```python
from build123d import *

# Parameters (mm, degrees)
F1_DEPTH = 3.175
F2_R     = 2.54
F3_DEPTH = 12.7
F4_R     = 1.1938
F5_DEPTH = 2.54


with BuildPart() as f1:
    # F0 (on Top) → F1 (new body)
    with BuildSketch(Plane.XY):
        with BuildLine():
            Line((32.885008, 3.175), (0, 3.175))
            ThreePointArc((0, 3.175), (-3.175, 0), (0, -3.175))
            Line((0, -3.175), (32.885008, -3.175))
            ThreePointArc((32.885008, -3.175), (36.060008, 0), (32.885008, 3.175))
        make_face()
    extrude(amount=F1_DEPTH)

    # F2 (on face) → F3 (join)
    with BuildSketch(Plane.XY.offset(3.175)):
        with Locations((1.6764, 0)):
            Circle(F2_R)
    extrude(amount=F3_DEPTH)

    # F4 (on face) → F5 (join)
    with BuildSketch(Plane(origin=(0, 0, 0), x_dir=(1, 0, 0), z_dir=(0, 0, -1))):
        with Locations((13.335, 0)):
            Circle(F4_R)
        with Locations((29.845, 0)):
            Circle(F4_R)
    extrude(amount=F5_DEPTH)


solid = f1.part
```
Design review of the part built by this model. Coordinates are the model's own, in mm. A direction names the side the tool comes from. Give positions to 0.01 mm unless a question says otherwise; leave off trailing zeros. Loops run counter-clockwise (first coordinate to the right, second up) from the corner with the lowest first, then second, coordinate; pieces in that order, holes last. Notation, with made-up numbers: M 23.5,24 L 39.5,24 A23 ccw 39.5,37 Z; hole C 60.25,-4.75 d9. An arc over 180 degrees is marked long. Return JSON: item names as keys, results as strings. Group by question number.
Item 1: Mouldability with a two-part tool opening along X and no side actions: class faces 4 (the cylindrical face through (-3.174, 0.07, 1.565)), 5 (the flat face through (2, 0, 15.875)), 6 (the cylindrical face through (36.06, -0.07, 1.57)), 7 (the cylindrical face through (12.142, -0.052, -1.252)) as released by +X, released by -X, zero draft, split by the parting line, or undercut.
Item 2: We need section A-A (y = 0). Give the boundary of the cut face in (x, z) (3 decimals).
Item 3: Insertion check: pin 1 Ø1 at (y, z) = (1, 7.5) entering from +X; pin 2 Ø1 at (x, y) = (16, 0) entering from -Z; pin 3 Ø2 at (y, z) = (1.5, 7.5) entering from -X; pin 4 Ø1.5 at (x, z) = (7.5, 4) entering from +Y. Each pin has a flat end and moves straight along its axis. Give the tip position at first contact, or say it passes through.
Item 4: Tool access review of faces 1 (the cylindrical face through (4.1, 0.76, 9.44)), 2 (the cylindrical face through (30.984, -0.359, -1.252)), 3 (the flat face through (17, 3.175, 2)): name each direction out of +Z, -Z, +X, -X, +Y, -Y from which nothing blocks a thin tool from reaching the whole face with its end or side.
Item 5: We need section B-B (z = 14.25). Give the boundary of the cut face in (x, y).
Item 6: We need section D-D (y = 2). Give the boundary of the cut face in (x, z) (3 decimals).
Item 7: For probe 1 along X at (y, z) = (0, -1.5); probe 2 along Z at (x, y) = (8, 1.75) (3 decimals); probe 3 along Z at (x, y) = (2, -1.25) (3 decimals), list the stretches that pass through material, from the lowest coordinate up.
Item 8: We need section C-C (x = 8.5). Give the boundary of the cut face in (y, z) (3 decimals).
Output:
{
 "1": {"face 4": "released by -X", "face 5": "zero draft", "face 6": "released by +X", "face 7": "undercut"},
 "2": {"outline": "M -3.175,0 L 12.141,0 L 12.141,-2.54 L 14.529,-2.54 L 14.529,0 L 28.651,0 L 28.651,-2.54 L 31.039,-2.54 L 31.039,0 L 36.06,0 L 36.06,3.175 L 4.216,3.175 L 4.216,15.875 L -0.864,15.875 L -0.864,3.175 L -3.175,3.175 Z"},
 "3": {"pin 1": "stops at x = 4.17", "pin 2": "stops at z = 0", "pin 3": "stops at x = -0.81", "pin 4": "passes through"},
 "4": {"face 1": "+Z", "face 2": "-Z", "face 3": "+Z, -Z, +X, -X, +Y"},
 "5": {"outline": "C 1.68,0 d5.08"},
 "6": {"outline": "M -2.466,0 L 35.351,0 L 35.351,3.175 L 3.242,3.175 L 3.242,15.875 L 0.111,15.875 L 0.111,3.175 L -2.466,3.175 Z"},
 "7": {"probe 1": "x = 12.14 to 14.53, 28.65 to 31.04", "probe 2": "z = 0 to 3.175", "probe 3": "z = 0 to 15.875"},
 "8": {"outline": "M -3.175,0 L 3.175,0 L 3.175,3.175 L -3.175,3.175 Z"}
}
